Check sheet for the modelled part. Datum: model origin and axes. Units: mm. A direction names the side the tool comes from. Round coordinates to 2 decimals unless told otherwise and drop trailing zeros. Write each loop counter-clockwise with the first axis right and the second up, starting at its lowest first coordinate (ties: lowest second). Pieces come first, ordered by that corner, then holes. Notation, with made-up numbers: M 6.5,-14 L 61.5,-14 A18 ccw 61.5,16 Z; hole C 30,89.5 d4. An arc over 180 degrees is marked long. Answer in a Markdown table with one row per item.
```python
from build123d import *

# Parameters (mm, degrees)
SKETCH1_W           = 30
SKETCH1_H           = 93.98
BOSS_EXTRUDE1_DEPTH = 12
FILLET1_R           = 8
SKETCH2_R           = 4
CUT_EXTRUDE1_DEPTH  = 8
SKETCH3_R           = 1.5
CUT_EXTRUDE2_DEPTH  = 31
SKETCH4_R           = 2
CUT_EXTRUDE3_DEPTH  = 2.5


with BuildPart() as part:
    # Sketch1 → Boss-Extrude1 (new body)
    with BuildSketch(Plane.XY):
        Rectangle(SKETCH1_W, SKETCH1_H)
    extrude(amount=BOSS_EXTRUDE1_DEPTH)

    # Fillet1
    fillet1_edges = [part.edges().sort_by_distance(p)[0] for p in [
        (15, -46.99, 6),
        (-15, -46.99, 6),
        (-15, 46.99, 6),
        (15, 46.99, 6),
    ]]
    fillet(fillet1_edges, radius=FILLET1_R)

    # Sketch2 → Cut-Extrude1 (cut)
    with BuildSketch(Plane.XY.offset(12)):
        with Locations((0, 7.99)):
            Circle(SKETCH2_R)
        with Locations((0, 34.49)):
            Circle(SKETCH2_R)
        with Locations((0, -34.494880812)):
            Circle(SKETCH2_R)
    extrude(amount=-CUT_EXTRUDE1_DEPTH, mode=Mode.SUBTRACT)

    # Sketch3 → Cut-Extrude2 (cut, through all)
    with BuildSketch(Plane.ZY.offset(15)):
        with Locations((7, 34.49)):
            Circle(SKETCH3_R)
        with Locations((7, 7.99)):
            Circle(SKETCH3_R)
        with Locations((7, -34.494880812)):
            Circle(SKETCH3_R)
    extrude(amount=-CUT_EXTRUDE2_DEPTH, mode=Mode.SUBTRACT)

    # Sketch4 → Cut-Extrude3 (cut)
    with BuildSketch(Plane(origin=(0, 0, 0), x_dir=(-1, 0, 0), z_dir=(0, 0, -1))):
        with Locations((0, -26.99)):
            Circle(SKETCH4_R)
        with Locations((0, 26.99)):
            Circle(SKETCH4_R)
    extrude(amount=-CUT_EXTRUDE3_DEPTH, mode=Mode.SUBTRACT)


solid = part.part
```
1. Section check A-A, the plane y = 7.99. Record the cut outline in (x, z), and give its area (3 significant figures).
Found:
| item | result |
|---|---|
| outline | M -15,0 L 15,0 L 15,5.5 L 4,5.5 L 4,4 L -4,4 L -4,5.5 L -15,5.5 Z; M -15,8.5 L -4,8.5 L -4,12 L -15,12 Z; M 4,8.5 L 15,8.5 L 15,12 L 4,12 Z |
| area | 230 mm2 |
2. Section check B-B, the plane z = 6.5. Count the separate pieces of the cut face and the enclosed holes in it, and give its area (3 significant figures).
Found:
| item | result |
|---|---|
| separate pieces | 4 |
| enclosed holes | 0 |
| area | 2,430 mm2 |
3. Go/stop test with flat-tipped pins: pin 1 (3 mm diameter, centred on x = 0, y = 26.99, fed in from -Z); pin 2 (6 mm diameter, centred on x = 12, z = 3.5, fed in from +Y). Record where each tip stops, or that it passes through.
Found:
| item | result |
|---|---|
| pin 1 | stops at z = 2.5 |
| pin 2 | stops at y = 46.74 |
4. Draft check along Z on faces 1 (the face through (9.28, 8.06, 5.5)), 2 (the face through (9.28, 33.58, 5.81)), 3 (the face through (12.719, 44.584, 6.084)), 4 (the face through (0, 1, 0)). Enter one of: +Z half, -Z half, draft (parallel to the pull), parting line (faces both ways), or undercut.
Found:
| item | result |
|---|---|
| face 1 | undercut |
| face 2 | undercut |
| face 3 | draft |
| face 4 | -Z half |
5. Section check D-D, the plane x = -5. Record the cut outline in (y, z), and give its area (3 significant figures).
Found:
| item | result |
|---|---|
| outline | M -46.99,0 L 46.99,0 L 46.99,12 L -46.99,12 Z; hole C -34.49,7 d3; hole C 7.99,7 d3; hole C 34.49,7 d3 |
| area | 1,110 mm2 |
6. Section check C-C, the plane x = 0. Record the cut outline in (y, z).
Found:
| item | result |
|---|---|
| outline | M -46.99,0 L -28.99,0 L -28.99,2.5 L -24.99,2.5 L -24.99,0 L 24.99,0 L 24.99,2.5 L 28.99,2.5 L 28.99,0 L 46.99,0 L 46.99,12 L 38.49,12 L 38.49,4 L 30.49,4 L 30.49,12 L 11.99,12 L 11.99,4 L 3.99,4 L 3.99,12 L -30.49,12 L -30.49,4 L -38.49,4 L -38.49,12 L -46.99,12 Z |
7. Scan lines: L1, parallel to Y at x = 0, z = 10; L2, parallel to X at y = 7.99, z = 9.75; L3, parallel to Y at x = -6.5, z = 7. Record each from-to range of solid material in increasing order.
Found:
| item | result |
|---|---|
| L1 | y = -46.99 to -38.49, -30.49 to 3.99, 11.99 to 30.49, 38.49 to 46.99 |
| L2 | x = -15 to -4, 4 to 15 |
| L3 | y = -46.99 to -35.99, -32.99 to 6.49, 9.49 to 32.99, 35.99 to 46.99 |
8. Access from +Z, -Z, +X, -X, +Y, -Y to the whole of each face (thin tool, end or side, straight path). Record for faces 5 (the face through (3.695, 32.958, 8.056)), 6 (the face through (0.434, -28.942, 1.232)), 7 (the face through (-12.719, 44.584, 6.084)).
Found:
| item | result |
|---|---|
| face 5 | +Z |
| face 6 | -Z |
| face 7 | +Z, -Z, -X, +Y |
